Read the model definition and answer for the solid it produces. Units are mm, in the model's axes. A direction names the side the tool comes from. Coordinates: 2 decimals unless noted, no trailing zeros. Order: outer loops, then holes, each group sorted by start corner. A loop starts at its lowest first (then second) coordinate and runs counter-clockwise, first axis right, second up. Notation, with made-up numbers: M 20.5,73 L 34.5,73 A19 cw 34.5,105 Z; hole C 55,5.25 d10. An arc over 180 degrees is marked long. Write each question's results on one line, items separated by ' | '.
```python
from build123d import *

# Parameters (mm, degrees)
SKETCH1_W           = 9.9
SKETCH1_H           = 6
BOSS_EXTRUDE1_DEPTH = 7.7
SKETCH2_W           = 6.3
SKETCH2_H           = 4.6
CUT_EXTRUDE1_DEPTH  = 5
SKETCH3_W           = 1.1
SKETCH3_H           = 6
CUT_EXTRUDE2_DEPTH  = 4.4
SKETCH4_W           = 3.6
SKETCH4_H           = 0.7
CUT_EXTRUDE3_DEPTH  = 5
SKETCH5_W           = 7.7
SKETCH5_H           = 0.9
CUT_EXTRUDE4_DEPTH  = 4.4
SKETCH6_W           = 0.5
SKETCH6_H           = 0.5
BOSS_EXTRUDE2_DEPTH = 3.7


with BuildPart() as part:
    # Sketch1 → Boss-Extrude1 (new body)
    with BuildSketch(Plane(origin=(0, 0, 0), x_dir=(1, 0, 0), z_dir=(0, 1, 0))):
        Rectangle(SKETCH1_W, SKETCH1_H)
    extrude(amount=BOSS_EXTRUDE1_DEPTH)

    # Sketch2 → Cut-Extrude1 (cut)
    with BuildSketch(Plane(origin=(0, 7.7, 0), x_dir=(1, 0, 0), z_dir=(0, 1, 0))):
        Rectangle(SKETCH2_W, SKETCH2_H)
    extrude(amount=-CUT_EXTRUDE1_DEPTH, mode=Mode.SUBTRACT)

    # Sketch3 → Cut-Extrude2 (cut)
    with BuildSketch(Plane(origin=(0, 7.7, 0), x_dir=(1, 0, 0), z_dir=(0, 1, 0))):
        with Locations((-4.4, 0)):
            Rectangle(SKETCH3_W, SKETCH3_H)
        with Locations((4.4, 0)):
            Rectangle(SKETCH3_W, SKETCH3_H)
    extrude(amount=-CUT_EXTRUDE2_DEPTH, mode=Mode.SUBTRACT)

    # Sketch4 → Cut-Extrude3 (cut)
    with BuildSketch(Plane(origin=(0, 7.7, 0), x_dir=(1, 0, 0), z_dir=(0, 1, 0))):
        with Locations((0, -2.65)):
            Rectangle(SKETCH4_W, SKETCH4_H)
    extrude(amount=-CUT_EXTRUDE3_DEPTH, mode=Mode.SUBTRACT)

    # Sketch5 → Cut-Extrude4 (cut)
    with BuildSketch(Plane(origin=(0, 7.7, 0), x_dir=(1, 0, 0), z_dir=(0, 1, 0))):
        with Locations((0, -1.85)):
            Rectangle(SKETCH5_W, SKETCH5_H)
    extrude(amount=-CUT_EXTRUDE4_DEPTH, mode=Mode.SUBTRACT)

    # Sketch6 → Boss-Extrude2 (add)
    with BuildSketch(Plane(origin=(0, 2.7, 0), x_dir=(1, 0, 0), z_dir=(0, 1, 0))):
        with Locations((-1.175, -1.15)):
            Rectangle(SKETCH6_W, SKETCH6_H)
        with Locations((1.175, -1.15)):
            Rectangle(SKETCH6_W, SKETCH6_H)
    extrude(amount=BOSS_EXTRUDE2_DEPTH)


solid = part.part
```
(1) The part is cut by section B-B, the plane y = 7. Write down the section's boundary in (x, z).
Conclusion:
outline: M -3.85,-3 L 3.85,-3 L 3.85,1.4 L 3.15,1.4 L 3.15,-2.3 L -3.15,-2.3 L -3.15,1.4 L -3.85,1.4 Z; M -3.85,2.3 L -1.8,2.3 L -1.8,3 L -3.85,3 Z; M 1.8,2.3 L 3.85,2.3 L 3.85,3 L 1.8,3 Z
(2) Straight lines are drawn through the part: line 1 (X direction, y = 5.5, z = -1.25); line 2 (Z direction, x = -3.5, y = 6). For each, find the intervals that lie inside material, in ascending order.
Conclusion:
line 1: -3.85 to -3.15, 3.15 to 3.85 | line 2: -3 to 1.4, 2.3 to 3
(3) The part is cut by section C-C, the plane x = 3.5. Write down the section's boundary in (y, z).
Conclusion:
outline: M 0,-3 L 7.7,-3 L 7.7,1.4 L 3.3,1.4 L 3.3,2.3 L 7.7,2.3 L 7.7,3 L 0,3 Z
(4) The mould has two halves that part along Z. Classify faces 1 (the flat face through (0, 4, -3)), 2 (the flat face through (-3.85, 6, -1)), 3 (the flat face through (-3.15, 5, 0)), 4 (the flat face through (0, 2, 3)): pulls with the +Z half, pulls with the -Z half, needs draft (parallel to the pull), parting line crosses it, or undercut.
Conclusion:
face 1: pulls with the -Z half | face 2: needs draft | face 3: undercut | face 4: pulls with the +Z half
(5) The part is cut by section A-A, the plane y = 5.5. Write down the section's boundary in (x, z) (3 decimals).
Conclusion:
outline: M -3.85,-3 L 3.85,-3 L 3.85,1.4 L 3.15,1.4 L 3.15,-2.3 L -3.15,-2.3 L -3.15,1.4 L -3.85,1.4 Z; M -3.85,2.3 L -1.8,2.3 L -1.8,3 L -3.85,3 Z; M -1.425,0.9 L -0.925,0.9 L -0.925,1.4 L -1.425,1.4 Z; M 0.925,0.9 L 1.425,0.9 L 1.425,1.4 L 0.925,1.4 Z; M 1.8,2.3 L 3.85,2.3 L 3.85,3 L 1.8,3 Z
(6) The part is cut by section D-D, the plane z = 0.35. Write down the section's boundary in (x, y), then the cut area to 4 significant figures.
Conclusion:
outline: M -4.95,0 L 4.95,0 L 4.95,3.3 L 3.85,3.3 L 3.85,7.7 L 3.15,7.7 L 3.15,2.7 L -3.15,2.7 L -3.15,7.7 L -3.85,7.7 L -3.85,3.3 L -4.95,3.3 Z | area: 35.05 mm²
(7) Given pin 1 (0.6 mm diameter, centred on y = 5, z = 1, fed in from +X); pin 2 (2.5 mm diameter, centred on x = 0.5, z = -1, fed in from +Y); pin 3 (0.6 mm diameter, centred on x = 1, y = 4.5, fed in from +Z), each flat-ended and moving along its own axis, determine where each tip first touches the part or whether it passes through.
Conclusion:
pin 1: x = 3.85 | pin 2: y = 2.7 | pin 3: z = 1.4
(8) For faces 5 (the flat face through (0, 5, -2.3)), 6 (the flat face through (3.85, 6, -1)), 7 (the flat face through (0, 0, 0)), determine the directions among +Z, -Z, +X, -X, +Y, -Y from which every point of the face is accessible in a straight line to the end or side of a thin tool.
Conclusion:
face 5: +Y | face 6: +Z, -Z, +X, +Y | face 7: +Z, -Z, +X, -X, -Y
